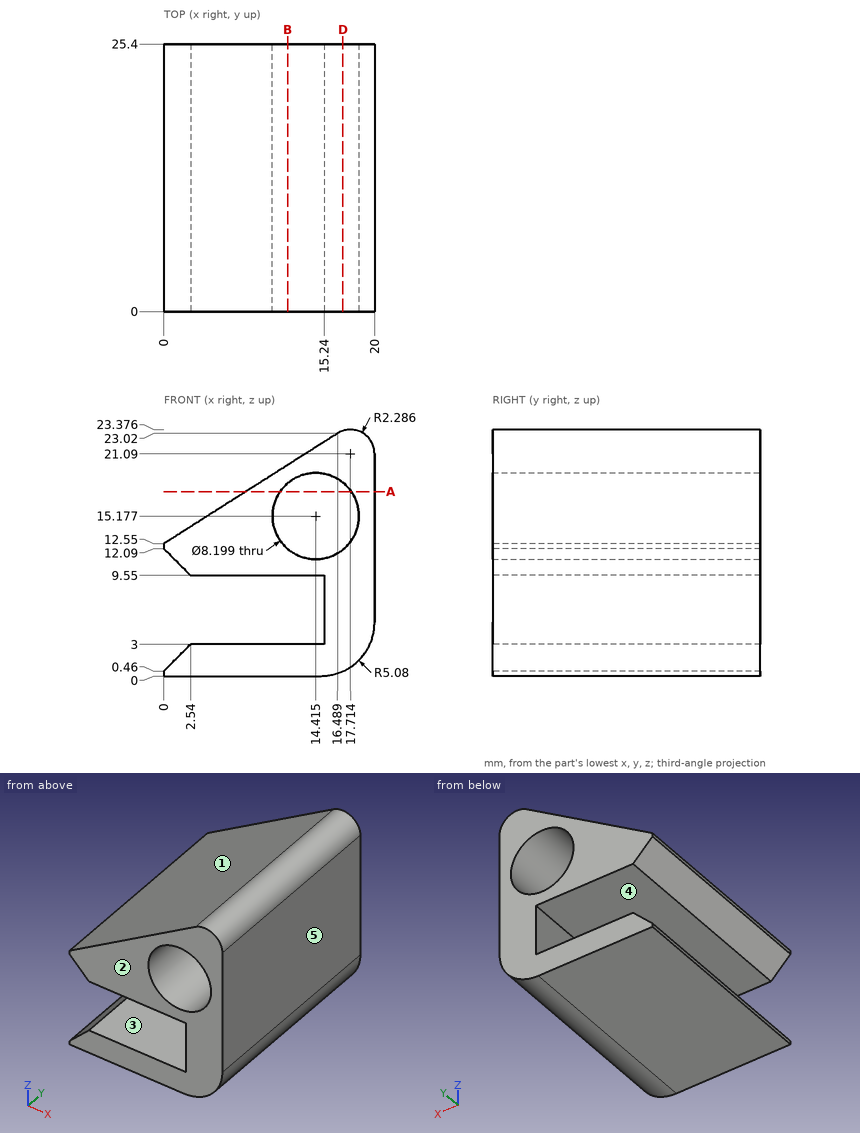
Here's the drawing with two shaded views (mm, measured from the low corner). I have some questions. A direction names the side the tool comes from. Coordinates: 2 decimals unless noted, no trailing zeros. Loops run counter-clockwise (first coordinate to the right, second up) from the corner with the lowest first, then second, coordinate; pieces in that order, holes last. Notation, with made-up numbers: M -6.75,5.5 L 9.25,5.5 A30 cw 9.25,38.5 Z; hole C 74,-37.75 d10. An arc over 180 degrees is marked long. Put each result on its own line as item: value. Start each with the question number.
(1) Imagine slicing it at B-B on x = 11.75. List the corners of the cut face in (y, z) for me.
(2) Which directions (+Z, -Z, +X, -X, +Y, -Y) give clear straight access to the entire face, cutting with the end or side of a thin tool? Please do the marked faces 4 and 5.
(3) Imagine slicing it at D-D on x = 17. List the corners of the cut face in (y, z) for me (1 decimal), and give its area (3 significant figures).
(4) We'd pull the mould along Z, two halves only. Please class the marked faces 1, 2 and 3: +Z half, -Z half, draft (parallel to the pull), parting line (faces both ways), or undercut.
(5) I need wall thicknesses on probe 1 along Z at (x, y) = (4.25, 6.25); probe 2 along Z at (x, y) = (8.5, 2); probe 3 along X at (y, z) = (18.5, 8). Which ranges of each line are inside material? Lowest first, please.
(6) Imagine slicing it at A-A on z = 17.5. List the corners of the cut face in (x, y) for me (1 decimal).
(7) Will these pins go through, and if not, where does the flat tip stop? pin 1 Ø3 at (x, z) = (7, 20.5) entering from -Y; pin 2 Ø1.5 at (y, z) = (20.5, 3.5) entering from +X; pin 3 Ø2 at (y, z) = (7.5, 6) entering from -X; pin 4 Ø4 at (x, y) = (6, 6.5) entering from +Z.
Worked answers:
1. outline: M 0,0 L 25.4,0 L 25.4,3 L 0,3 Z; M 0,9.55 L 25.4,9.55 L 25.4,12.06 L 0,12.06 Z; M 0,18.29 L 25.4,18.29 L 25.4,20.01 L 0,20.01 Z
2. face 4: -X, +Y, -Y
2. face 5: +Z, -Z, +X, +Y, -Y
3. outline: M 0,0.4 L 25.4,0.4 L 25.4,12 L 0,12 Z; M 0,18.4 L 25.4,18.4 L 25.4,23.3 L 0,23.3 Z
3. area: 418 mm2
4. face 1: +Z half
4. face 2: draft
4. face 3: undercut
5. probe 1: z = 0 to 3, 9.55 to 15.25
5. probe 2: z = 0 to 3, 9.55 to 17.95
5. probe 3: x = 15.24 to 20
6. outline: M 7.8,0 L 11,0 L 11,25.4 L 7.8,25.4 Z; M 17.8,0 L 20,0 L 20,25.4 L 17.8,25.4 Z
7. pin 1: passes through
7. pin 2: stops at x = 19.93
7. pin 3: stops at x = 15.24
7. pin 4: stops at z = 17.63
